Work out the finished part from the listing and answer in its coordinate system (mm). A direction names the side the tool comes from. Round coordinates to 2 decimals unless told otherwise and drop trailing zeros. Loops run counter-clockwise (first coordinate to the right, second up) from the corner with the lowest first, then second, coordinate; pieces in that order, holes last. Notation, with made-up numbers: M 21.25,85 L 25.25,85 A35 cw 25.25,120 Z; hole C 72,-1 d5. An arc over 180 degrees is marked long. One line per item, written item: value.
Autodesk Inventor part; units mm, degrees
ref_plane "YZ Plane" through (0, 0, 0) normal (1, 0, 0) x (0, 1, 0)
ref_plane "XZ Plane" through (0, 0, 0) normal (0, 1, 0) x (-1, 0, 0)
ref_plane "XY Plane" through (0, 0, 0) normal (0, 0, 1) x (1, 0, 0)
sketch "Sketch1" plane through (0, 0, 0) normal (0, 0, 1) x (1, 0, 0)
  circle A0 centre (0, 0) radius 4.7625
  circle A1 centre (0, 0) radius 11.1125
  circle A2 centre (0, 0) radius 12.6873
  circle A3 centre (0, 0) radius 5.715
  circle A4 centre (0, 0) radius 10.16
  dimension "d0" = 9.525
  dimension "d1" = 22.225
  dimension "d2" = 25.3746
  dimension "d7" = 20.32
  dimension "d8" = 11.43
extrude "Extrusion1" add sketch "Sketch1" along normal blind 7.112 contours A1 | A3 | A4
extrude "Extrusion2" add sketch "Sketch1" along normal blind 1.5748 contours A2
extrude "Extrusion3" cut sketch "Sketch1" along normal blind 0.635 contours A4
sketch "Sketch2" plane through (0, 0, 7.112) normal (0, 0, 1) x (1, 0, 0)
  circle A0 centre (0, 0) radius 5.715
  circle A1 centre (0, 0) radius 10.16
extrude "Extrusion4" cut sketch "Sketch2" against normal blind 0.635
properties part number ".375 ID .875 OD bearing"
1) Find the intervals of material crossed by probe 1 along Y at (x, z) = (0, 0.2) (1 decimal); probe 2 along Y at (x, z) = (0, 6.6) (1 decimal); probe 3 along Y at (x, z) = (0, 3.75), in increasing order. Write a range as from..to.
Check values:
probe 1: -12.7..-10.2, -5.7..-4.8, 4.8..5.7, 10.2..12.7
probe 2: -11.1..-10.2, -5.7..-4.8, 4.8..5.7, 10.2..11.1
probe 3: -11.11..-4.76, 4.76..11.11
2) Each of these flat-tipped pins is pushed along its axis until it touches: pin 1 (4 mm diameter, centred on y = -10, z = 1, fed in from +X); pin 2 (3 mm diameter, centred on y = -8.5, z = 6, fed in from -X); pin 3 (1 mm diameter, centred on x = -1.5, z = 6, fed in from -Y). Where does it stop, or does it pass through?
Check values:
pin 1: x = 9.85
pin 2: x = -8.63
pin 3: y = -11.07
3) Find section D-D (y = -6.5). Give the vertices of the cut face in (x, z) (3 decimals), then the cut area to 3 significant figures.
Check values:
outline: M -10.896,0 L -7.809,0 L -7.809,0.635 L 7.809,0.635 L 7.809,0 L 10.896,0 L 10.896,1.575 L 9.013,1.575 L 9.013,7.112 L 7.809,7.112 L 7.809,6.477 L -7.809,6.477 L -7.809,7.112 L -9.013,7.112 L -9.013,1.575 L -10.896,1.575 Z
area: 114 mm2
4) The mould has two halves that part along Y. Classify faces 1 (the face through (4.6, -10.3, 1.575)), 2 (the face through (5.45, -1.72, 0.31)), 3 (the face through (10.6, -3.34, 4.3)): +Y half, -Y half, draft (parallel to the pull), parting line (faces both ways), or undercut.
Check values:
face 1: draft
face 2: undercut
face 3: parting line
5) Find section A-A (y = 0). Give the vertices of the cut face in (x, z) (1 decimal), then the cut area to 3 significant figures.
Check values:
outline: M -12.7,0 L -10.2,0 L -10.2,0.6 L -5.7,0.6 L -5.7,0 L -4.8,0 L -4.8,7.1 L -5.7,7.1 L -5.7,6.5 L -10.2,6.5 L -10.2,7.1 L -11.1,7.1 L -11.1,1.6 L -12.7,1.6 Z; M 4.8,0 L 5.7,0 L 5.7,0.6 L 10.2,0.6 L 10.2,0 L 12.7,0 L 12.7,1.6 L 11.1,1.6 L 11.1,7.1 L 10.2,7.1 L 10.2,6.5 L 5.7,6.5 L 5.7,7.1 L 4.8,7.1 Z
area: 84.0 mm2
6) For faces 4 (the face through (-1.323, 10.074, 6.799)), 5 (the face through (10, -3, 7.112)), 6 (the face through (4.4, -4.4, 0.635)), determine the directions among +Z, -Z, +X, -X, +Y, -Y from which every point of the face is accessible in a straight line to the end or side of a thin tool.
Check values:
face 4: +Z
face 5: +Z, +X, -X, +Y, -Y
face 6: -Z
7) Find section C-C (z = 4.5). Give the vertices of the cut face in (x, y) (1 decimal), then the cut area to 3 significant figures.
Check values:
outline: C 0,0 d22.2; hole C 0,0 d9.5
area: 317 mm2
